Check sheet for the modelled part. Datum: model origin and axes. Units: mm. A direction names the side the tool comes from. Coordinates: 2 decimals unless noted, no trailing zeros. Write each loop counter-clockwise with the first axis right and the second up, starting at its lowest first coordinate (ties: lowest second). Pieces come first, ordered by that corner, then holes. Notation, with made-up numbers: (60, -17) -> (105, -17) arc R11 cw to (105, -5) -> close; hole circle Ø8 at (50.25, 17). An arc over 180 degrees is marked (long way). Put each result on its own line as item: value.
```python
from build123d import *

# Parameters (mm, degrees)
CROQUIS2_W                = 2.5
CROQUIS2_H                = 29
CROQUIS2_R                = 0.8
SALIENTE_EXTRUIR2_DEPTH   = 2
TALADRO_ROSCADO_M41_D     = 3.3
TALADRO_ROSCADO_M41_DEPTH = 11.5
TALADRO_ROSCADO_M41_TIP   = 0.991420021


with BuildPart() as part:
    # Croquis2 → Saliente-Extruir2 (new body)
    with BuildSketch(Plane(origin=(0, 0, 0), x_dir=(1, 0, 0), z_dir=(0, 1, 0))):
        with BuildLine():
            Line((-69.290093462, 11.720598128), (-71.290093462, 11.720598128))
            Line((-71.290093462, 11.720598128), (-71.290093462, -52.279401872))
            Line((-71.290093462, -52.279401872), (-55.290093462, -52.279401872))
            ThreePointArc((-55.290093462, -52.279401872), (-23.290093462, -20.279401872), (-55.290093462, 11.720598128))
            Line((-55.290093462, 11.720598128), (-69.290093462, 11.720598128))
        make_face()
        with Locations((-61.073318824, -19.453109229)):
            Rectangle(CROQUIS2_W, CROQUIS2_H, mode=Mode.SUBTRACT)
        with Locations((-56.754226246, -18.397495979)):
            Circle(CROQUIS2_R, mode=Mode.SUBTRACT)
        Polygon((-57.823318824, -16.953109229), (-57.823318824, -4.953109229), (-52.823318824, -4.953109229), (-52.823318824, -22.953109229), (-55.323318824, -22.953109229), (-55.323318824, -16.953109229), align=None, mode=Mode.SUBTRACT)
    extrude(amount=SALIENTE_EXTRUIR2_DEPTH)

    # Taladro roscado M41
    with Locations(Plane(origin=(0, 2, 0), x_dir=(1, 0, 0), z_dir=(0, 1, 0))):
        with Locations((-51.290093462, 5.720598128), (-51.290093462, -46.279401872)):
            Hole(TALADRO_ROSCADO_M41_D / 2, depth=TALADRO_ROSCADO_M41_DEPTH)
            with Locations((0, 0, -(TALADRO_ROSCADO_M41_DEPTH + TALADRO_ROSCADO_M41_TIP / 2))):  # 118° drill point
                Cone(0, TALADRO_ROSCADO_M41_D / 2, TALADRO_ROSCADO_M41_TIP, mode=Mode.SUBTRACT)


solid = part.part
```
Q1. Material ranges on line 1 along Z through (x, y) = (-54.5, 0.3); line 2 along Z through (x, y) = (-61, 1.15); line 3 along Z through (x, y) = (-50.5, 0.35), recorded low to high.
Recorded:
line 1: z = -11.71 to 4.95, 22.95 to 52.27
line 2: z = -11.72 to 4.95, 33.95 to 52.28
line 3: z = -11.36 to -7.17, -4.27 to 44.83, 47.73 to 51.92
Q2. Cross-section at B-B (y = 1.5). Record the cut outline in (x, z).
Recorded:
outline: (-71.29, -11.72) -> (-55.29, -11.72) arc R32 ccw to (-55.29, 52.28) -> (-71.29, 52.28) -> close; hole (-62.32, 4.95) -> (-59.82, 4.95) -> (-59.82, 33.95) -> (-62.32, 33.95) -> close; hole (-57.82, 4.95) -> (-52.82, 4.95) -> (-52.82, 22.95) -> (-55.32, 22.95) -> (-55.32, 16.95) -> (-57.82, 16.95) -> close; hole circle Ø1.6 at (-56.75, 18.4); hole circle Ø3.3 at (-51.29, -5.72); hole circle Ø3.3 at (-51.29, 46.28)
Q3. Mould release check, pull along X, two halves, no side actions. Record for faces 3 (the cylindrical face through (-23.3, 1, 21)), 4 (the cylindrical face through (-55.99, 0.99, 18.16)), 5 (the flat face through (-71.29, 1, 20)), 6 (the flat face through (-63, 1, -11.721)): released by +X, released by -X, zero draft, split by the parting line, or undercut.
Recorded:
face 3: released by +X
face 4: undercut
face 5: released by -X
face 6: zero draft
Q4. Cross-section at C-C (x = -31). Record the cut outline in (y, z).
Recorded:
outline: (0, -0.55) -> (2, -0.55) -> (2, 41.11) -> (0, 41.11) -> close
Q5. Tool access check on faces 1 (the flat face through (-52.823, 1, 14)), 2 (the flat face through (-63, 1, 52.279)). Record the directions out of +Z, -Z, +X, -X, +Y, -Y that give a thin tool (end or side, any length) a straight path to the whole face; none if there is none.
Recorded:
face 1: +Y, -Y
face 2: +Z, +X, -X, +Y, -Y
Q6. Cross-section at A-A (z = 7). Record the cut outline in (x, y), plus the area to 3 significant figures.
Recorded:
outline: (-71.29, 0) -> (-62.32, 0) -> (-62.32, 2) -> (-71.29, 2) -> close; (-59.82, 0) -> (-57.82, 0) -> (-57.82, 2) -> (-59.82, 2) -> close; (-52.82, 0) -> (-26.18, 0) -> (-26.18, 2) -> (-52.82, 2) -> close
area: 75.2 mm2
Q7. Cross-section at D-D (z = 21.5). Record the cut outline in (x, y), plus the area to 3 significant figures.
Recorded:
outline: (-71.29, 0) -> (-62.32, 0) -> (-62.32, 2) -> (-71.29, 2) -> close; (-59.82, 0) -> (-55.32, 0) -> (-55.32, 2) -> (-59.82, 2) -> close; (-52.82, 0) -> (-23.31, 0) -> (-23.31, 2) -> (-52.82, 2) -> close
area: 86.0 mm2
Q8. Depth check by flat-ended pin: P1, Ø0.6, axis at x = -54.5, y = 0.5, coming from the -Z side; P2, Ø4, axis at x = -34, z = 42.5, coming from the -Y side; P3, Ø1, axis at x = -56.75, z = 18.4, coming from the -Y side; P4, Ø1, axis at y = 0.5, z = 17.5, coming from the +X side. Enter the tip coordinate at first touch or a pass-through.
Recorded:
P1: stops at z = -11.72
P2: stops at y = 0
P3: passes through
P4: stops at x = -23.37
